from build123d import *

# Parameters (mm, degrees)
F0_W     = 23.495
F0_H     = 12.7
F1_DEPTH = 1.5875
F2_R     = 1.5875
F3_DEPTH = 25.4
F4_W     = 23.495
F4_H     = 3.175
F5_DEPTH = 76.2
F7_R     = 1.5875
F8_DEPTH = 25.4


with BuildPart() as f1:
    # F0 (on Front) → F1 (new body)
    with BuildSketch(Plane.XZ):
        Rectangle(F0_W, F0_H)
    extrude(amount=F1_DEPTH)

    # F2 (on face) → F3 (cut)
    with BuildSketch(Plane.XZ.offset(1.5875)):
        with Locations((-5.87375, -3.175)):
            Circle(F2_R)
        with Locations((5.87375, -3.175)):
            Circle(F2_R)
    extrude(amount=-F3_DEPTH, mode=Mode.SUBTRACT)

    # F4 (on face) → F5 (join)
    with BuildSketch(Plane.XZ.offset(1.5875)):
        with Locations((0, 4.7625)):
            Rectangle(F4_W, F4_H)
    extrude(amount=F5_DEPTH)

    # F6: F1 across face


with BuildPart() as f1_1:
    add(f1.part)
    add(f1.part.mirror(Plane(origin=(0, -77.7875, 4.7625), x_dir=(1, 0, 0), z_dir=(0, -1, 0))))

    # F7 (on face) → F8 (cut)
    with BuildSketch(Plane.XY.offset(6.35)):
        with Locations((0, -34.032031)):
            Circle(F7_R)
        with Locations((0, -24.308594)):
            Circle(F7_R)
        with Locations((0, -131.266406)):
            Circle(F7_R)
        with Locations((0, -121.542969)):
            Circle(F7_R)
    extrude(amount=-F8_DEPTH, mode=Mode.SUBTRACT)


solid = f1_1.part
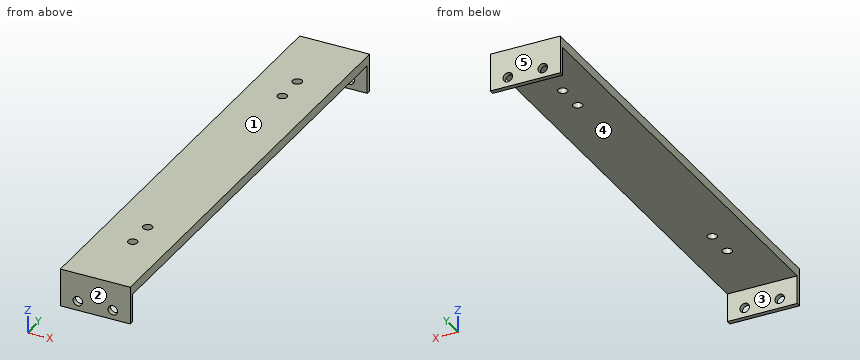
The listing builds one solid part. Answer for the finished solid, in the listing's coordinates (mm). Face numbers are marked on the shaded views. A direction names the side the tool comes from. Coordinates: 2 decimals unless noted, no trailing zeros. Write each question's results on one line, items separated by ' | '.
Item 1: The part is cut by section A-A on x = 0. State how many separate pieces and enclosed holes the cut face has, and give its area (3 significant figures).
Answer below:
separate pieces: 5 | enclosed holes: 0 | area: 484 mm2
Item 2: Which of the six approach directions +Z, -Z, +X, -X, +Y, -Y give full straight-line access (tool end or side, diameter ignored) to the marked faces 4 and 5?
Answer below:
face 4: -Z, +X, -X | face 5: +Z, -Z, +X, -X, +Y
Item 3: Consider probe 1 along Y at (x, z) = (0, 4.1) (3 decimals); probe 2 along Y at (x, z) = (2.75, 2.75) (1 decimal); probe 3 along Z at (x, y) = (2.5, -91) (3 decimals). Determine where each line is inside the solid, lowest interval first. Write a range as [from, to].
Answer below:
probe 1: [-155.575, -132.854], [-129.679, -123.13], [-119.955, -35.62], [-32.445, -25.896], [-22.721, 0] | probe 2: [-155.6, -154], [-1.6, 0] | probe 3: [3.175, 6.35]
Item 4: Given P1, Ø5, axis at x = -5.87, z = -3.18, coming from the -Y side (3 decimals); P2, Ø12, axis at x = 3.5, y = -46.5, coming from the -Z side (3 decimals), each flat-ended and moving along its own axis, determine where each tip first touches the part or whether it passes through.
Answer below:
P1: y = -155.575 | P2: z = 3.175
Item 5: For a pull along Y with two mould halves and no side action, classify the marked faces 1, 2 and 3 as released by +Y, released by -Y, zero draft, split by the parting line, or undercut.
Answer below:
face 1: zero draft | face 2: released by -Y | face 3: undercut
